Part model, mm, in its own coordinate system. A direction names the side the tool comes from. Give positions to 0.01 mm unless a question says otherwise; leave off trailing zeros. Order: outer loops, then holes, each group sorted by start corner. A loop starts at its lowest first (then second) coordinate and runs counter-clockwise, first axis right, second up.
1. Which spindle directions (+Z, -Z, +X, -X, +Y, -Y) get a long thin tool onto all of the face, cutting with end or side? Do faces 1 (the flat face through (3.175, 50, 1)), 2 (the flat face through (113, -1, 101.6)). Say none if no direction does.
2. Slice it at A-A on z = -51. List the corners of the cut face in (x, y) (3 decimals), and give its area (3 significant figures).
3. Slice it at C-C on x = 48.5. List the corners of the cut face in (y, z) (3 decimals), and give its area (3 significant figures).
4. Drop flat-ended pins along their axis: pin 1 Ø2 at (y, z) = (20, 64) entering from +X (3 decimals); pin 2 Ø8 at (x, z) = (179.5, 15) entering from +Y. Give the stop position or say it passes through.
5. Probe line 1 (X direction, y = 25, z = 92) (3 decimals); line 2 (Y direction, x = 131, z = -82) (3 decimals). List the from-to ranges inside material, lowest first.
6. Slice it at B-B on y = 40.5. List the corners of the cut face in (x, z) (3 decimals), and give its area (3 significant figures).
from build123d import *

# Parameters (mm, degrees)
SKETCH1_W           = 3.175
SKETCH1_H           = 98.425
BOSS_EXTRUDE1_DEPTH = 101.6
CHAMFER1_SIZE       = 5.08


with BuildPart() as part:
    # Sketch1 → Boss-Extrude1 (new, symmetric)
    with BuildSketch(Plane.XY):
        Polygon((3.175, 0), (0, 0), (0, -3.175), (228.6, -3.175), (228.6, 0), (5.715, 0), align=None)
        with Locations((1.5875, 49.2125)):
            Rectangle(SKETCH1_W, SKETCH1_H)
        with BuildLine():
            Line((3.175, 2.54), (3.175, 0))
            Line((3.175, 0), (5.715, 0))
            ThreePointArc((5.715, 0), (3.918948776, 0.743948776), (3.175, 2.54))
        make_face()
    extrude(amount=BOSS_EXTRUDE1_DEPTH, both=True)

    # Chamfer1
    # the kernel refuses this chamfer: 5.08 mm, written as the material it takes off along each edge
    with BuildSketch(Plane(origin=(228.6, 0, 114.664149579), x_dir=(-0.9996219169112968, 0.027495876610586324, 0), z_dir=(0, 0, -1))) as chamfer1_piece_1:
        Polygon((CHAMFER1_SIZE * 0.999621916911, -CHAMFER1_SIZE * 0.0274958766106), (-CHAMFER1_SIZE * 0.0274958766106, -CHAMFER1_SIZE * 0.999621916911), (0, 0), align=None)
    extrude(amount=229.328299158, mode=Mode.SUBTRACT)


solid = part.part
Data:
1. face 1: +Z, -Z, +X, +Y
1. face 2: +Z, +X, -X, +Y, -Y
2. outline: (0, -3.175) - (226.695, -3.175) - (223.52, 0) - (5.715, 0) arc R2.54 cw to (3.175, 2.54) - (3.175, 98.425) - (0, 98.425) - close
2. area: 1,030 mm2
3. outline: (-3.175, -101.6) - (0, -101.6) - (0, 101.6) - (-3.175, 101.6) - close
3. area: 645 mm2
4. pin 1: stops at x = 3.175
4. pin 2: stops at y = 0
5. line 1: x = 0 to 3.175
5. line 2: y = -3.175 to 0
6. outline: (0, -101.6) - (3.175, -101.6) - (3.175, 101.6) - (0, 101.6) - close
6. area: 645 mm2
